from build123d import *

# Parameters (mm, degrees)
SKETCH_R    = 4
PAD_DEPTH   = 6.35
SKETCH001_R = 1.25
HOLE_DEPTH  = 10
HOLE_TIPS_R = 1.25


with BuildPart() as part:
    # Sketch → Pad (new body, symmetric)
    with BuildSketch(Plane.XZ):
        with BuildLine():
            Line((-15, -7.62744), (-15, 40))
            Line((-15, 40), (15, 40))
            Line((15, 7.627403), (15, 40))
            Line((15, 7.627403), (27.491385, -4.863982))
            Line((27.491385, -4.863982), (27.491385, -7.863982))
            Line((27.491385, -7.863982), (21.920307, -13.435044))
            Line((15.605634, -7.120352), (21.920307, -13.435044))
            ThreePointArc((15.605634, -7.120352), (7.120352, -7.12034), (7.12034, -15.605621))
            Line((7.12034, -15.605621), (13.435014, -21.920313))
            Line((13.435014, -21.920313), (7.863944, -27.491383))
            Line((7.863944, -27.491383), (4.863944, -27.491383))
            Line((4.863944, -27.491383), (-15, -7.62744))
        make_face()
        Circle(SKETCH_R, mode=Mode.SUBTRACT)
    extrude(amount=PAD_DEPTH, both=True)

    # Sketch001 (on Face7 of Pad) → Hole (cut)
    with BuildSketch(Plane(origin=(0, 0, 40), x_dir=(-1, 0, 0), z_dir=(0, 0, 1))):
        with Locations((-10, 0)):
            Circle(SKETCH001_R)
        with Locations((10, 0)):
            Circle(SKETCH001_R)
    extrude(amount=-HOLE_DEPTH, mode=Mode.SUBTRACT)

    # Hole tips → Hole tip 1 section 0
    with BuildSketch(Plane(origin=(0, 0, 30), x_dir=(-1, 0, 0), z_dir=(0, 0, 1)), mode=Mode.PRIVATE) as hole_tip_1_s0:
        with Locations((-10, 0)):
            Circle(HOLE_TIPS_R)
    loft([hole_tip_1_s0.sketch, Vertex(10, 0, 29.248924)], mode=Mode.SUBTRACT)

    # Hole tips → Hole tip 2 section 0
    with BuildSketch(Plane(origin=(0, 0, 30), x_dir=(-1, 0, 0), z_dir=(0, 0, 1)), mode=Mode.PRIVATE) as hole_tip_2_s0:
        with Locations((10, 0)):
            Circle(HOLE_TIPS_R)
    loft([hole_tip_2_s0.sketch, Vertex(-10, 0, 29.248924)], mode=Mode.SUBTRACT)


solid = part.part
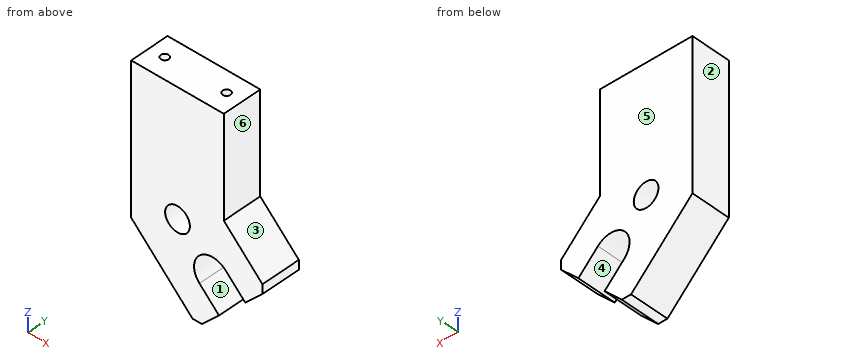
Source: CAD feature listing. Evaluate the final solid. Frame: model axes, mm. Face numbers are marked on the shaded views. A direction names the side the tool comes from. Coordinates: 2 decimals unless noted, no trailing zeros. Order: outer loops, then holes, each group sorted by start corner. A loop starts at its lowest first (then second) coordinate and runs counter-clockwise, first axis right, second up. Notation, with made-up numbers: M 87.5,64 L 105.5,64 A31 cw 105.5,92 Z; hole C 85.5,83.5 d3. An arc over 180 degrees is marked long. Write each question's results on one line, items separated by ' | '. Start each with the question number.
1. Reachability of the marked faces 4, 5 and 6 from +Z, -Z, +X, -X, +Y, -Y: full face, straight path, thin tool, end or side. Return the list, or none.
2. Section D-D, the plane z = 0. Return the cut outline in (x, y).
3. Section B-B, the plane z = 32.5. Return the cut outline in (x, y).
4. Draft query along Z for the marked faces 1, 2 and 3. Return one class per face: +Z half, -Z half, draft (parallel to the pull), parting line (faces both ways), or undercut.
5. Section C-C, the plane x = 0. Return the cut outline in (y, z).
6. Section A-A, the plane y = -2.5. Return the cut outline in (x, z).
7. Material intervals for L1, parallel to X at y = 0, z = 32.25; L2, parallel to X at y = 0.5, z = 24.5; L3, parallel to Z at x = -2, y = -0.5, sorted ascending.
8. Pin query (flat end, axial travel): pin 1 (6.5 mm diameter, centred on y = -1.5, z = 26, fed in from +X); pin 2 (1 mm diameter, centred on x = 14, y = 3.5, fed in from -Z); pin 3 (9 mm diameter, centred on x = 0, z = 0, fed in from -Y); pin 4 (1.5 mm diameter, centred on x = 10, y = 0, fed in from +Z). Return the tip coordinate at first contact, or that it passes through.
Solution:
1) face 4: -Z, +Y, -Y | face 5: +Z, -Z, +X, -X, +Y | face 6: +Z, +X, +Y, -Y
2) outline: M -15,-6.35 L -4,-6.35 L -4,6.35 L -15,6.35 Z; M 4,-6.35 L 22.63,-6.35 L 22.63,6.35 L 4,6.35 Z
3) outline: M -15,-6.35 L 15,-6.35 L 15,6.35 L -15,6.35 Z; hole C -10,0 d2.5; hole C 10,0 d2.5
4) face 1: undercut | face 2: draft | face 3: +Z half
5) outline: M -6.35,-22.63 L 6.35,-22.63 L 6.35,-4 L -6.35,-4 Z; M -6.35,4 L 6.35,4 L 6.35,40 L -6.35,40 Z
6) outline: M -15,-7.63 L 4.86,-27.49 L 7.86,-27.49 L 13.44,-21.92 L 7.12,-15.61 A6 cw 15.61,-7.12 L 21.92,-13.44 L 27.49,-7.86 L 27.49,-4.86 L 15,7.63 L 15,40 L -15,40 Z; hole C 0,0 d8
7) L1: -15 to -11.25, -8.75 to 8.75, 11.25 to 15 | L2: -15 to 15 | L3: -20.63 to -3.46, 3.46 to 40
8) pin 1: x = 15 | pin 2: z = -6.25 | pin 3: y = -6.35 | pin 4: z = 29.7
